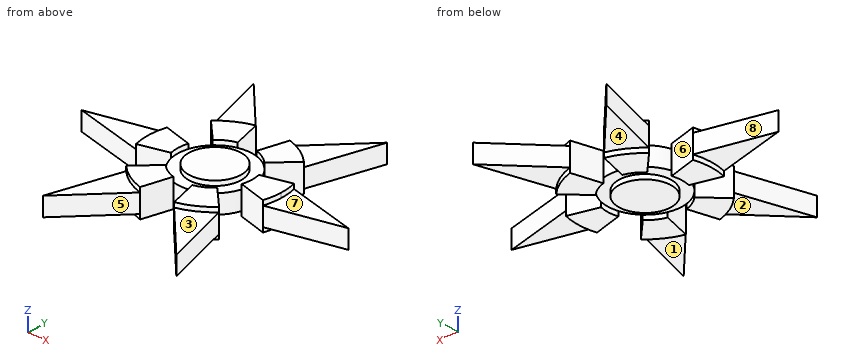
from build123d import *

# Parameters (mm, degrees)
SKETCH1_R             = 14
BOSS_EXTRUDE1_DEPTH   = 7.5
BOSS_EXTRUDE1_2_DEPTH = 7.5
BOSS_EXTRUDE1_3_DEPTH = 7.5
BOSS_EXTRUDE1_4_DEPTH = 7.5
BOSS_EXTRUDE1_5_DEPTH = 7.5
BOSS_EXTRUDE1_6_DEPTH = 7.5
BOSS_EXTRUDE1_7_DEPTH = 7.5
SKETCH1_3_R           = 20
SKETCH1_3_R_2         = 14
BOSS_EXTRUDE2_DEPTH   = 5


with BuildPart() as part:
    # Sketch1 → Boss-Extrude1 (new, symmetric)
    with BuildSketch(Plane.XY):
        Circle(SKETCH1_R)
    extrude(amount=BOSS_EXTRUDE1_DEPTH, both=True)



with BuildPart() as body_2:
    # Sketch1 → Boss-Extrude1 2 (new, symmetric)
    with BuildSketch(Plane.XY):
        with BuildLine():
            Line((-5.176380902, 19.318516526), (-9.317485624, 34.773329746))
            ThreePointArc((-9.317485624, 34.773329746), (-18, 31.176914536), (-25.455844123, 25.455844123))
            Line((-25.455844123, 25.455844123), (-14.142135624, 14.142135624))
            ThreePointArc((-14.142135624, 14.142135624), (-10, 17.320508076), (-5.176380902, 19.318516526))
        make_face()
    extrude(amount=BOSS_EXTRUDE1_2_DEPTH, both=True)


with BuildPart() as body_3:
    # Sketch1 → Boss-Extrude1 3 (new, symmetric)
    with BuildSketch(Plane.XY):
        with BuildLine():
            Line((14.142135624, 14.142135624), (25.455844123, 25.455844123))
            ThreePointArc((25.455844123, 25.455844123), (18, 31.176914536), (9.317485624, 34.773329746))
            Line((9.317485624, 34.773329746), (5.176380902, 19.318516526))
            ThreePointArc((5.176380902, 19.318516526), (10, 17.320508076), (14.142135624, 14.142135624))
        make_face()
    extrude(amount=BOSS_EXTRUDE1_3_DEPTH, both=True)


with BuildPart() as body_4:
    # Sketch1 → Boss-Extrude1 4 (new, symmetric)
    with BuildSketch(Plane.XY):
        with BuildLine():
            Line((-19.318516526, 5.176380902), (-34.773329746, 9.317485624))
            ThreePointArc((-34.773329746, 9.317485624), (-36, 0), (-34.773329746, -9.317485624))
            Line((-34.773329746, -9.317485624), (-19.318516526, -5.176380902))
            ThreePointArc((-19.318516526, -5.176380902), (-20, 0), (-19.318516526, 5.176380902))
        make_face()
    extrude(amount=BOSS_EXTRUDE1_4_DEPTH, both=True)


with BuildPart() as body_5:
    # Sketch1 → Boss-Extrude1 5 (new, symmetric)
    with BuildSketch(Plane.XY):
        with BuildLine():
            ThreePointArc((36, 0), (35.692015009, 4.69894292), (34.773329746, 9.317485624))
            Line((34.773329746, 9.317485624), (19.318516526, 5.176380902))
            ThreePointArc((19.318516526, 5.176380902), (19.828897227, 2.610523844), (20, 0))
            ThreePointArc((20, 0), (19.828897227, -2.610523844), (19.318516526, -5.176380902))
            Line((19.318516526, -5.176380902), (34.773329746, -9.317485624))
            ThreePointArc((34.773329746, -9.317485624), (35.692015009, -4.69894292), (36, 0))
        make_face()
    extrude(amount=BOSS_EXTRUDE1_5_DEPTH, both=True)


with BuildPart() as body_6:
    # Sketch1 → Boss-Extrude1 6 (new, symmetric)
    with BuildSketch(Plane.XY):
        with BuildLine():
            ThreePointArc((9.317485624, -34.773329746), (18, -31.176914536), (25.455844123, -25.455844123))
            Line((25.455844123, -25.455844123), (14.142135624, -14.142135624))
            ThreePointArc((14.142135624, -14.142135624), (10, -17.320508076), (5.176380902, -19.318516526))
            Line((5.176380902, -19.318516526), (9.317485624, -34.773329746))
        make_face()
    extrude(amount=BOSS_EXTRUDE1_6_DEPTH, both=True)


with BuildPart() as body_7:
    # Sketch1 → Boss-Extrude1 7 (new, symmetric)
    with BuildSketch(Plane.XY):
        with BuildLine():
            ThreePointArc((-25.455844123, -25.455844123), (-18, -31.176914536), (-9.317485624, -34.773329746))
            Line((-9.317485624, -34.773329746), (-5.176380902, -19.318516526))
            ThreePointArc((-5.176380902, -19.318516526), (-10, -17.320508076), (-14.142135624, -14.142135624))
            Line((-14.142135624, -14.142135624), (-25.455844123, -25.455844123))
        make_face()
    extrude(amount=BOSS_EXTRUDE1_7_DEPTH, both=True)


with BuildPart() as part_1:
    add(part.part)

    add(body_2.part)  # Boss-Extrude2 merges body 2

    add(body_3.part)  # Boss-Extrude2 merges body 3

    add(body_4.part)  # Boss-Extrude2 merges body 4

    add(body_5.part)  # Boss-Extrude2 merges body 5

    add(body_6.part)  # Boss-Extrude2 merges body 6

    add(body_7.part)  # Boss-Extrude2 merges body 7
    # Sketch1_3 → Boss-Extrude2 (add, symmetric)
    # profile 1 of 7: a face of its own
    with BuildSketch(Plane.XY):
        with BuildLine():
            ThreePointArc((-25.455844123, 25.455844123), (-18, 31.176914536), (-9.317485624, 34.773329746))
            Line((-9.317485624, 34.773329746), (-36.5, 63.219854476))
            Line((-36.5, 63.219854476), (-25.455844123, 25.455844123))
        make_face()
    # profile 2 of 7: a face of its own
    with BuildSketch(Plane.XY):
        with BuildLine():
            ThreePointArc((9.317485624, 34.773329746), (18, 31.176914536), (25.455844123, 25.455844123))
            Line((25.455844123, 25.455844123), (36.5, 63.219854476))
            Line((36.5, 63.219854476), (9.317485624, 34.773329746))
        make_face()
    # profile 3 of 7: a face of its own
    with BuildSketch(Plane.XY):
        with BuildLine():
            Line((73, 0), (34.773329746, 9.317485624))
            ThreePointArc((34.773329746, 9.317485624), (35.692015009, 4.69894292), (36, 0))
            ThreePointArc((36, 0), (35.692015009, -4.69894292), (34.773329746, -9.317485624))
            Line((34.773329746, -9.317485624), (73, 0))
        make_face()
    # profile 4 of 7: a face of its own
    with BuildSketch(Plane.XY):
        with BuildLine():
            ThreePointArc((-34.773329746, -9.317485624), (-36, 0), (-34.773329746, 9.317485624))
            Line((-34.773329746, 9.317485624), (-73, 0))
            Line((-73, 0), (-34.773329746, -9.317485624))
        make_face()
    # profile 5 of 7: a face of its own
    with BuildSketch(Plane.XY):
        with BuildLine():
            Line((-36.5, -63.219854476), (-9.317485624, -34.773329746))
            ThreePointArc((-9.317485624, -34.773329746), (-18, -31.176914536), (-25.455844123, -25.455844123))
            Line((-25.455844123, -25.455844123), (-36.5, -63.219854476))
        make_face()
    # profile 6 of 7: a face of its own
    with BuildSketch(Plane.XY):
        with BuildLine():
            Line((36.5, -63.219854476), (25.455844123, -25.455844123))
            ThreePointArc((25.455844123, -25.455844123), (18, -31.176914536), (9.317485624, -34.773329746))
            Line((9.317485624, -34.773329746), (36.5, -63.219854476))
        make_face()
    # profile 7 of 7: a face of its own
    with BuildSketch(Plane.XY):
        Circle(SKETCH1_3_R)
        Circle(SKETCH1_3_R_2, mode=Mode.SUBTRACT)
    extrude(amount=BOSS_EXTRUDE2_DEPTH, both=True)


solid = part_1.part
Here's how the part is built. I have some questions about the finished solid (model axes, mm). Face numbers are marked on the shaded views. A direction names the side the tool comes from. Coordinates: 2 decimals unless noted, no trailing zeros. Loops run counter-clockwise (first coordinate to the right, second up) from the corner with the lowest first, then second, coordinate; pieces in that order, holes last.
1. Imagine slicing it at A-A, the plane x = -33. Please give me the cut outline in (y, z), and give its area (3 significant figures).
2. For the marked faces 1, 2, 3 and 4, which set-ups out of +Z, -Z, +X, -X, +Y, -Y let a thin tool reach every point of the face, with its end or its side?
3. If we mould it in two halves opening along X, with no side actions, what happens to the marked faces 5, 6, 7 and 8? For each: pulls with the +X half, pulls with the -X half, needs draft (parallel to the pull), parting line crosses it, or undercut.
4. Imagine slicing it at C-C, the plane y = 23. Please give me the cut outline in (x, z).
5. I need wall thicknesses on L1, parallel to Y at x = 21, z = -5.5; L2, parallel to X at y = 26, z = -2.25; L3, parallel to X at y = 24.5, z = 1.5. Which ranges of each line are inside material? Lowest first, please.
6. Imagine slicing it at D-D, the plane x = 0. Please give me the cut outline in (y, z).
7. For P1, Ø1.5, axis at x = 32, y = 40, coming from the -Z side; P2, Ø9.5, axis at x = 56, y = 1, coming from the +Z side; P3, Ø6, axis at x = 7, z = 1.5, coming from the +Y side; P4, Ø9.5, axis at x = -60.5, y = 2, coming from the -Z side, each with a flat end and sliding along its axis, tell me the tip position at first contact or that it passes through.
Taken from the geometry:
1. outline: (-59.56, -5) - (-51.25, -5) - (-51.25, 5) - (-59.56, 5) - close; (-8.84, -7.5) - (8.84, -7.5) - (8.84, 7.5) - (-8.84, 7.5) - close; (51.25, -5) - (59.56, -5) - (59.56, 5) - (51.25, 5) - close
1. area: 431 mm2
2. face 1: -Z, +X, -Y
2. face 2: -Z, -X, -Y
2. face 3: +Z, +X, -Y
2. face 4: -Z, -X, +Y
3. face 5: undercut
3. face 6: undercut
3. face 7: needs draft
3. face 8: pulls with the -X half
4. outline: (-23, -7.5) - (-6.16, -7.5) - (-6.16, 7.5) - (-23, 7.5) - close; (6.16, -7.5) - (23, -7.5) - (23, 7.5) - (6.16, 7.5) - close
5. L1: y = -29.24 to -21, -5.63 to 5.63, 21 to 29.24
5. L2: x = -25.61 to -6.97, 6.97 to 25.61
5. L3: x = -24.5 to -6.56, 6.56 to 24.5
6. outline: (-20, -5) - (-14, -5) - (-14, -7.5) - (14, -7.5) - (14, -5) - (20, -5) - (20, 5) - (14, 5) - (14, 7.5) - (-14, 7.5) - (-14, 5) - (-20, 5) - close
7. P1: passes through
7. P2: stops at z = 5
7. P3: stops at y = 35.49
7. P4: stops at z = -5
